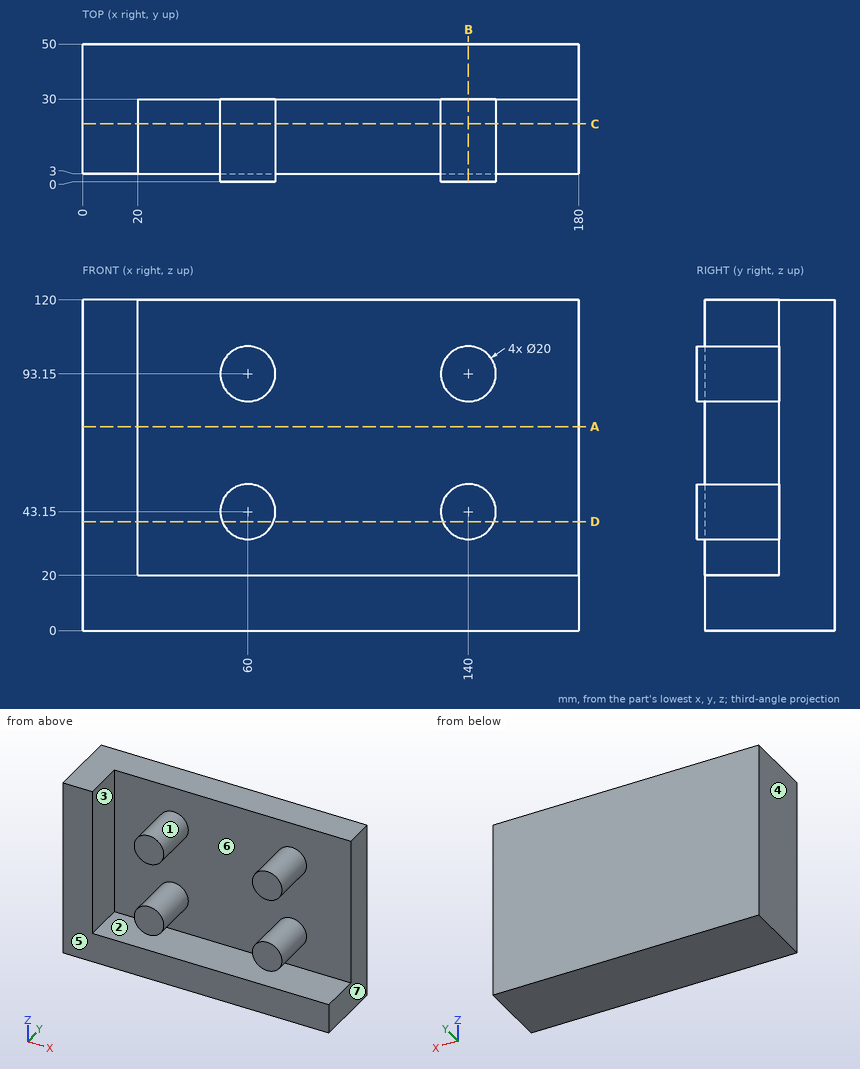
Verification items for this drawing (mm, ordinates from the low corner). A direction names the side the tool comes from. Give positions to 0.01 mm unless a question says otherwise; leave off trailing zeros. Write each loop counter-clockwise with the first axis right and the second up, starting at its lowest first coordinate (ties: lowest second). Pieces come first, ordered by that corner, then holes. Notation, with made-up numbers: (-11.5, 29.5) -> (24.5, 29.5) arc R20 cw to (24.5, 51.5) -> close; hole circle Ø8 at (86, -28.5). An arc over 180 degrees is marked (long way). Use CSV: the item, a comma, the result in double quotes. Start each with the question number.
Q1. Depth check by flat-ended pin: P1, Ø12, axis at x = 154.5, y = 17, coming from the +Z side; P2, Ø4, axis at x = 41.5, z = 33, coming from the -Y side; P3, Ø21.5, axis at x = 117.5, y = 13, coming from the +Z side. Enter the tip coordinate at first touch or a pass-through.
Q2. Cross-section at A-A on z = 74. Enter the section's corners in (x, y), and give its area (3 significant figures).
Q3. Cross-section at B-B on x = 140. Enter the section's corners in (y, z), and give its area (3 significant figures).
Q4. Scan lines: line 1 along X through (y, z) = (29, 43.5); line 2 along X through (y, z) = (28.5, 99.5) (1 decimal); line 3 along Y through (x, z) = (92.5, 39). Record each from-to range of solid material in increasing order.
Q5. Tool access check on the marked faces 1, 2 and 3. Record the directions out of +Z, -Z, +X, -X, +Y, -Y that give a thin tool (end or side, any length) a straight path to the whole face; none if there is none.
Q6. Release check for a two-part mould opening along X. For the marked faces 4, 5, 6 and 7 record: +X half, -X half, draft (parallel to the pull), parting line (faces both ways), or undercut.
Q7. Cross-section at C-C on y = 21. Enter the section's corners in (x, z).
Q8. Cross-section at D-D on z = 39.5. Enter the section's corners in (x, y), and give its area (3 significant figures).
Working result:
1,P1,"stops at z = 98.42"
1,P2,"stops at y = 30"
1,P3,"stops at z = 20"
2,outline,"(0, 3) -> (20, 3) -> (20, 30) -> (180, 30) -> (180, 50) -> (0, 50) -> close"
2,area,"4,140 mm^2"
3,outline,"(0, 33.15) -> (30, 33.15) -> (30, 20) -> (3, 20) -> (3, 0) -> (50, 0) -> (50, 120) -> (30, 120) -> (30, 103.15) -> (0, 103.15) -> (0, 83.15) -> (30, 83.15) -> (30, 53.15) -> (0, 53.15) -> close"
3,area,"4,140 mm^2"
4,line 1,"x = 0 to 20, 50.01 to 69.99, 130.01 to 149.99"
4,line 2,"x = 0 to 20, 52.3 to 67.7, 132.3 to 147.7"
4,line 3,"y = 30 to 50"
5,face 1,"-Y"
5,face 2,"+X, -Y"
5,face 3,"+Z, -Y"
6,face 4,"-X half"
6,face 5,"draft"
6,face 6,"undercut"
6,face 7,"+X half"
7,outline,"(0, 0) -> (180, 0) -> (180, 20) -> (20, 20) -> (20, 120) -> (0, 120) -> close; circle Ø20 at (60, 43.15); circle Ø20 at (60, 93.15); circle Ø20 at (140, 43.15); circle Ø20 at (140, 93.15)"
8,outline,"(0, 3) -> (20, 3) -> (20, 30) -> (50.69, 30) -> (50.69, 0) -> (69.31, 0) -> (69.31, 30) -> (130.69, 30) -> (130.69, 0) -> (149.31, 0) -> (149.31, 30) -> (180, 30) -> (180, 50) -> (0, 50) -> close"
8,area,"5,260 mm^2"
